Geometry: final body of the model. Coordinates: model frame, mm. A direction names the side the tool comes from. Coordinates: 2 decimals unless noted, no trailing zeros. Write each loop counter-clockwise with the first axis right and the second up, starting at its lowest first coordinate (ties: lowest second). Pieces come first, ordered by that corner, then holes. Notation, with made-up numbers: M 73.25,-30 L 82.25,-30 A20 ccw 82.25,7 Z; hole C 8.25,17 d8. An arc over 180 degrees is marked long. Write item = value, one per line. Start each with the question number.
Item 1: Pull-direction query (X, two-part tool) for faces 1 (the cylindrical face through (8, -0.3, 12.5)), 2 (the flat face through (17, -19.932, 15)), 3 (the cylindrical face through (17.435, -0.381, -0.196)); classes: +X half, -X half, draft (parallel to the pull), parting line (faces both ways), or undercut.
Item 2: Section C-C on x = 0. Output: boundary loops of the cut face in (y, z).
Item 3: Ray query, L1, parallel to X at y = -19, z = -13; L2, parallel to Y at x = 15.5, z = -7; L3, parallel to X at y = -0.15, z = 0. Return the intervals inside material, ascending. Write a range as [from, to].
Item 4: Section B-B on z = 17. Output: boundary loops of the cut face in (x, y).
Item 5: First-contact query: pin 1 Ø1 at (x, z) = (-9.5, 6.5) entering from -Y; pin 2 Ø0.7 at (x, y) = (17, -9.5) entering from +Z; pin 3 Ø2 at (x, z) = (14, 9) entering from +Y; pin 4 Ø0.7 at (y, z) = (-0.5, 16.5) entering from +X. Flat tips, straight axial feed; report the tip coordinate or a pass-through.
Item 6: Reachability of faces 4 (the flat face through (-17.237, -12, 0)), 5 (the cylindrical face through (-8, -0.3, 12.5)) from +Z, -Z, +X, -X, +Y, -Y: full face, straight path, thin tool, end or side. Return the list, or none.
Item 7: Section A-A on y = -13.75. Output: boundary loops of the cut face in (x, z).
Item 8: Section D-D on z = 6. Output: boundary loops of the cut face in (x, y), plus the area to 3 significant figures.
from build123d import *

# Parameters (mm, degrees)
SKETCH1_W           = 33
SKETCH1_H           = 40
BASE_FLANGE1_DEPTH  = 0.6
CUT_EXTRUDE1_DEPTH  = 10
EDGE_FLANGE1_DEPTH  = 28
SKETCH21_R          = 9.5
CUT_EXTRUDE11_DEPTH = 10
EDGE_FLANGE2_DEPTH  = 2.068329304


# Sheet-metal steps are written as plain solids
with BuildPart() as part:
    # Sketch1 → Base-Flange1 (new body)
    with BuildSketch(Plane(origin=(0, 0, 0), x_dir=(1, 0, 0), z_dir=(0, 1, 0))):
        Rectangle(SKETCH1_W, SKETCH1_H)
    extrude(amount=-BASE_FLANGE1_DEPTH)

    # Sketch6 → Cut-Extrude1 (cut)
    with BuildSketch(Plane(origin=(0, 0, 0), x_dir=(1, 0, 0), z_dir=(0, 1, 0))):
        with BuildLine():
            Line((-9.5, 20), (-9.5, 14))
            ThreePointArc((-9.5, 14), (-8, 12.5), (-6.5, 14))
            Line((-6.5, 14), (-6.5, 20))
            Line((-6.5, 20), (-9.5, 20))
        make_face()
        with BuildLine():
            Line((6.5, 20), (6.5, 14))
            ThreePointArc((6.5, 14), (8, 12.5), (9.5, 14))
            Line((9.5, 14), (9.5, 20))
            Line((9.5, 20), (6.5, 20))
        make_face()
        with BuildLine():
            Line((9.5, -20), (9.5, -14))
            ThreePointArc((9.5, -14), (8, -12.5), (6.5, -14))
            Line((6.5, -14), (6.5, -20))
            Line((6.5, -20), (9.5, -20))
        make_face()
        with BuildLine():
            Line((-9.5, -20), (-6.5, -20))
            Line((-6.5, -20), (-6.5, -14))
            ThreePointArc((-6.5, -14), (-8, -12.5), (-9.5, -14))
            Line((-9.5, -14), (-9.5, -20))
        make_face()
    extrude(amount=-CUT_EXTRUDE1_DEPTH, mode=Mode.SUBTRACT)

    # Edge-Flange1 section (across the edge) → Edge-Flange1 (add)
    with BuildSketch(Plane(origin=(17.2366, -0.6, -14), x_dir=(-1, 0, 0), z_dir=(0, 0, 1))):
        with BuildLine():
            Line((-0.6, 0.7366), (-0.6, 21.4))
            Line((-0.6, 21.4), (0, 21.4))
            Line((0, 21.4), (0, 0.7366))
            ThreePointArc((0, 0.7366), (0.215745145, 0.215745145), (0.7366, 0))
            Line((0.7366, 0), (0.7366, -0.6))
            ThreePointArc((0.7366, -0.6), (-0.208518924, -0.208518924), (-0.6, 0.7366))
        make_face()
    edge_flange1 = extrude(amount=EDGE_FLANGE1_DEPTH)

    # Mirror1: Edge-Flange1 across plane
    add(edge_flange1.mirror(Plane(origin=(0, 0, 0), x_dir=(0, 0, 1), z_dir=(1, 0, 0))))

    # Sketch21 → Cut-Extrude11 (cut)
    with BuildSketch(Plane(origin=(0, 0, 0), x_dir=(1, 0, 0), z_dir=(0, 1, 0))):
        with Locations(Location((0, 0, 0), (0, 0, 270))):
            Circle(SKETCH21_R)
    extrude(amount=-CUT_EXTRUDE11_DEPTH, mode=Mode.SUBTRACT)

    # Edge-Flange2 section (across the edge) → Edge-Flange2 (add)
    with BuildSketch(Plane(origin=(17.2366, -22, 14.7366), x_dir=(0, 0, -1), z_dir=(0, 1, 0))):
        with BuildLine():
            Line((-0.6, 0.7366), (-0.6, 1.546122954))
            Line((-0.6, 1.546122954), (0, 1.546122954))
            Line((0, 1.546122954), (0, 0.7366))
            ThreePointArc((0, 0.7366), (0.215745145, 0.215745145), (0.7366, 0))
            Line((0.7366, 0), (0.7366, -0.6))
            ThreePointArc((0.7366, -0.6), (-0.208518924, -0.208518924), (-0.6, 0.7366))
        make_face()
    extrude(amount=EDGE_FLANGE2_DEPTH)


solid = part.part
Responses:
q1.face_1 = undercut
q1.face_2 = draft
q1.face_3 = +X half
q2.outline = M -0.6,-20 L 0,-20 L 0,-9.5 L -0.6,-9.5 Z; M -0.6,9.5 L 0,9.5 L 0,20 L -0.6,20 Z
q3.L1 = [-17.84, -17.24], [17.24, 17.84]
q3.L2 = [-0.6, 0]
q3.L3 = [-17.12, -9.5], [9.5, 17.12]
q4.outline = M -16.5,-0.6 L -9.5,-0.6 L -9.5,0 L -16.5,0 Z; M -6.5,-0.6 L 6.5,-0.6 L 6.5,0 L -6.5,0 Z; M 9.5,-0.6 L 16.5,-0.6 L 16.5,0 L 9.5,0 Z
q5.pin_1 = -0.6
q5.pin_2 = 14
q5.pin_3 = 0
q5.pin_4 = 16.5
q6.face_4 = +Z, -Z, -Y
q6.face_5 = +Z, +Y, -Y
q7.outline = M -17.84,-14 L -17.24,-14 L -17.24,14 L -17.84,14 Z; M 17.24,-14 L 17.84,-14 L 17.84,14 L 17.24,14 Z
q8.outline = M -17.84,-22 L -17.24,-22 L -17.24,-1.34 A0.74 cw -16.5,-0.6 L -7.37,-0.6 L -7.37,0 L -16.5,0 A1.34 ccw -17.84,-1.34 Z; M 7.37,-0.6 L 16.5,-0.6 A0.74 cw 17.24,-1.34 L 17.24,-22 L 17.84,-22 L 17.84,-1.34 A1.34 ccw 16.5,0 L 7.37,0 Z
q8.area = 37.7 mm²
